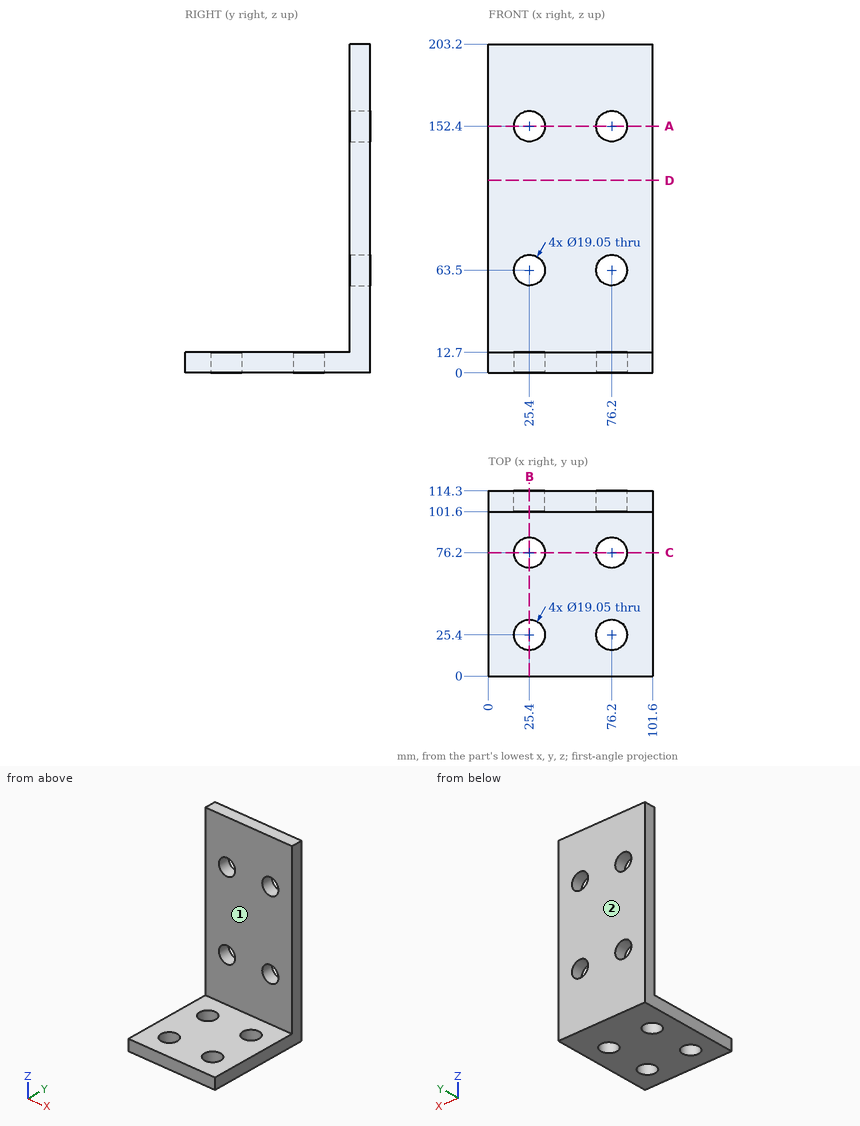
Could you check a few things on this drawing? It's one solid part, dimensions in mm from its lowest x, y, z. A direction names the side the tool comes from. Coordinates: 2 decimals unless noted, no trailing zeros. Loops run counter-clockwise (first coordinate to the right, second up) from the corner with the lowest first, then second, coordinate; pieces in that order, holes last.
1. Imagine slicing it at C-C (y = 76.2). Please give me the cut outline in (x, z) (3 decimals), and give its area (3 significant figures).
2. Imagine slicing it at A-A (z = 152.4). Please give me the cut outline in (x, y) (3 decimals).
3. I need wall thicknesses on L1, parallel to Y at x = 25.4, z = 4 (3 decimals); L2, parallel to X at y = 111, z = 63; L3, parallel to Z at x = 11, y = 26.5. Which ranges of each line are inside material? Lowest first, please.
4. For the marked faces 1 and 2, which set-ups out of +Z, -Z, +X, -X, +Y, -Y let a thin tool reach every point of the face, with its end or its side?
5. Imagine slicing it at D-D (z = 119). Please give me the cut outline in (x, y).
6. Imagine slicing it at B-B (x = 25.4). Please give me the cut outline in (y, z) (3 decimals).
7. For P1, Ø10, axis at x = 50, y = 53.5, coming from the +Z side; P2, Ø17, axis at x = 76.2, y = 25.4, coming from the -Z side; P3, Ø25, axis at x = 25.4, z = 152.4, coming from the -Y side, each with a flat end and sliding along its axis, tell me the tip position at first contact or that it passes through.
Computed values:
1. outline: (0, 0) - (15.875, 0) - (15.875, 12.7) - (0, 12.7) - close; (34.925, 0) - (66.675, 0) - (66.675, 12.7) - (34.925, 12.7) - close; (85.725, 0) - (101.6, 0) - (101.6, 12.7) - (85.725, 12.7) - close
1. area: 806 mm2
2. outline: (0, 101.6) - (15.875, 101.6) - (15.875, 114.3) - (0, 114.3) - close; (34.925, 101.6) - (66.675, 101.6) - (66.675, 114.3) - (34.925, 114.3) - close; (85.725, 101.6) - (101.6, 101.6) - (101.6, 114.3) - (85.725, 114.3) - close
3. L1: y = 0 to 15.875, 34.925 to 66.675, 85.725 to 114.3
3. L2: x = 0 to 15.89, 34.91 to 66.69, 85.71 to 101.6
3. L3: z = 0 to 12.7
4. face 1: +Z, +X, -X, -Y
4. face 2: +Z, -Z, +X, -X, +Y
5. outline: (0, 101.6) - (101.6, 101.6) - (101.6, 114.3) - (0, 114.3) - close
6. outline: (0, 0) - (15.875, 0) - (15.875, 12.7) - (0, 12.7) - close; (34.925, 0) - (66.675, 0) - (66.675, 12.7) - (34.925, 12.7) - close; (85.725, 0) - (114.3, 0) - (114.3, 53.975) - (101.6, 53.975) - (101.6, 12.7) - (85.725, 12.7) - close; (101.6, 73.025) - (114.3, 73.025) - (114.3, 142.875) - (101.6, 142.875) - close; (101.6, 161.925) - (114.3, 161.925) - (114.3, 203.2) - (101.6, 203.2) - close
7. P1: stops at z = 12.7
7. P2: passes through
7. P3: stops at y = 101.6
